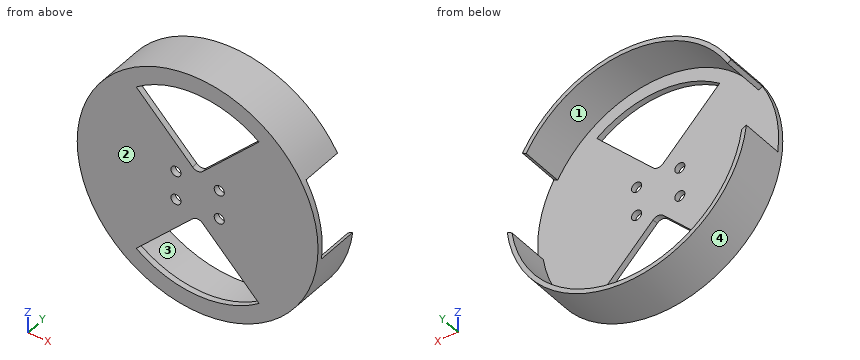
```python
from build123d import *

# Parameters (mm, degrees)
CROQUIS1_R              = 80.5
SALIENTE_EXTRUIR1_DEPTH = 4
CROQUIS2_R              = 83.5
CROQUIS2_R_2            = 80.5
EXTRUIR_L_MINA1_DEPTH   = 34
CORTAR_EXTRUIR1_START   = -30
CORTAR_EXTRUIR1_DEPTH   = 30
CORTAR_EXTRUIR3_DEPTH   = 4
CROQUIS6_R              = 3.5
CORTAR_EXTRUIR4_DEPTH   = 10


with BuildPart() as part:
    # Croquis1 → Saliente-Extruir1 (new body)
    with BuildSketch(Plane(origin=(0, 0, 0), x_dir=(1, 0, 0), z_dir=(0, 1, 0))):
        with Locations(Location((0, 0, 0), (0, 0, 270))):
            Circle(CROQUIS1_R)
    extrude(amount=SALIENTE_EXTRUIR1_DEPTH)

    # Croquis2 → Extruir-Lámina1 (add)
    with BuildSketch(Plane(origin=(0, 0, 0), x_dir=(1, 0, 0), z_dir=(0, 1, 0))):
        Circle(CROQUIS2_R)
        Circle(CROQUIS2_R_2, mode=Mode.SUBTRACT)
    extrude(amount=EXTRUIR_L_MINA1_DEPTH)

    # Croquis3 → Cortar-Extruir1 (cut)
    with BuildSketch(Plane(origin=(0, 34, 0), x_dir=(1, 0, 0), z_dir=(0, 1, 0)).offset(CORTAR_EXTRUIR1_START)):
        with BuildLine():
            Line((82.915347707, 9.8638286), (79.63686942, 11.756658922))
            ThreePointArc((79.63686942, 11.756658922), (80.283927371, 5.894150138), (80.5, 0))
            ThreePointArc((80.5, 0), (77.757029016, -20.834933131), (69.715045005, -40.25))
            Line((69.715045005, -40.25), (72.313121216, -41.75))
            ThreePointArc((72.313121216, -41.75), (80.654806495, -21.611390266), (83.5, 0))
            ThreePointArc((83.5, 0), (83.353708776, 4.940570133), (82.915347707, 9.8638286))
        make_face()
        with BuildLine():
            ThreePointArc((-69.715045005, -40.25), (-79.073837194, -15.085697577), (-79.63686942, 11.756658922))
            Line((-79.63686942, 11.756658922), (-82.915347707, 9.8638286))
            ThreePointArc((-82.915347707, 9.8638286), (-81.792213668, -16.801303023), (-72.313121216, -41.75))
            Line((-72.313121216, -41.75), (-69.715045005, -40.25))
        make_face()
    extrude(amount=CORTAR_EXTRUIR1_DEPTH, mode=Mode.SUBTRACT)

    # Croquis4 → Cortar-Extruir3 (cut)
    with BuildSketch(Plane.XZ):
        with BuildLine():
            Line((-42.603387144, 57.603387144), (-3.535533906, 18.535533906))
            ThreePointArc((-3.535533906, 18.535533906), (0, 17.071067812), (3.535533906, 18.535533906))
            Line((3.535533906, 18.535533906), (42.603387144, 57.603387144))
            ThreePointArc((42.603387144, 57.603387144), (0, 71.646345383), (-42.603387144, 57.603387144))
        make_face()
        with BuildLine():
            Line((-3.535533906, -18.535533906), (-42.603387144, -57.603387144))
            ThreePointArc((-42.603387144, -57.603387144), (0, -71.646345383), (42.603387144, -57.603387144))
            Line((42.603387144, -57.603387144), (3.535533906, -18.535533906))
            ThreePointArc((3.535533906, -18.535533906), (0, -17.071067812), (-3.535533906, -18.535533906))
        make_face()
    extrude(amount=-CORTAR_EXTRUIR3_DEPTH, mode=Mode.SUBTRACT)

    # Croquis6 → Cortar-Extruir4 (cut)
    with BuildSketch(Plane.XZ):
        with Locations(Location((-15, 10, 0), (0, 0, 270))):
            Circle(CROQUIS6_R)
        with Locations(Location((-15, -10, 0), (0, 0, 270))):
            Circle(CROQUIS6_R)
        with Locations(Location((15, 10, 0), (0, 0, 270))):
            Circle(CROQUIS6_R)
        with Locations(Location((15, -10, 0), (0, 0, 270))):
            Circle(CROQUIS6_R)
    extrude(amount=-CORTAR_EXTRUIR4_DEPTH, mode=Mode.SUBTRACT)


solid = part.part
```
CAD build for the part. Positions are in the model's coordinates, mm. Face numbers are marked on the shaded views. Give positions to 0.01 mm unless a question says otherwise; leave off trailing zeros. Loops run counter-clockwise (first coordinate to the right, second up) from the corner with the lowest first, then second, coordinate; pieces in that order, holes last. Notation, with made-up numbers: (-39.5, -20.5) -> (-6.5, -20.5) arc R13 ccw to (-6.5, -16.5) -> close; hole circle Ø11 at (3, -15). An arc over 180 degrees is marked (long way). Use a Markdown table: item, result.
1. Wall check: L1, parallel to X at y = 2.15, z = 10; L2, parallel to Y at x = -21.5, z = 33.5; L3, parallel to Z at x = -36, y = 16. Give the ranges that are in metal, low to high. Write a range as [from, to].
Check result:
| item | result |
|---|---|
| L1 | x = [-82.9, -18.5], [-11.5, 11.5], [18.5, 82.9] |
| L2 | y = [0, 4] |
| L3 | z = [-75.34, -72], [72, 75.34] |
2. Flat gauge pins, fed straight in: pin 1 (8 mm diameter, centred on y = 22, z = -58, fed in from +X); pin 2 (1 mm diameter, centred on x = -38.5, y = 6.5, fed in from +Z); pin 3 (5.5 mm diameter, centred on x = 15, z = -10, fed in from +Y); pin 4 (8 mm diameter, centred on x = -15, z = -10, fed in from +Y). Where does each tip first touch, or does it go through?
Check result:
| item | result |
|---|---|
| pin 1 | stops at x = 63.69 |
| pin 2 | stops at z = 74.35 |
| pin 3 | passes through |
| pin 4 | stops at y = 4 |
3. Slice it at B-B (x = 0). List the corners of the cut face in (y, z).
Check result:
| item | result |
|---|---|
| outline | (0, -83.5) -> (34, -83.5) -> (34, -80.5) -> (4, -80.5) -> (4, -71.65) -> (0, -71.65) -> close; (0, -17.07) -> (4, -17.07) -> (4, 17.07) -> (0, 17.07) -> close; (0, 71.65) -> (4, 71.65) -> (4, 80.5) -> (34, 80.5) -> (34, 83.5) -> (0, 83.5) -> close |
4. Slice it at C-C (z = -55). List the corners of the cut face in (x, y).
Check result:
| item | result |
|---|---|
| outline | (-62.83, 0) -> (-40, 0) -> (-40, 4) -> (-58.78, 4) -> (-58.78, 34) -> (-62.83, 34) -> close; (40, 0) -> (62.83, 0) -> (62.83, 34) -> (58.78, 34) -> (58.78, 4) -> (40, 4) -> close |
5. Slice it at A-A (y = 19). List the corners of the cut face in (x, z), plus the area to 3 significant figures.
Check result:
| item | result |
|---|---|
| outline | (-82.92, -9.86) arc R83.5 ccw to (82.92, -9.86) -> (79.64, -11.76) arc R80.5 cw to (-79.64, -11.76) -> close; (-72.31, 41.75) -> (-69.72, 40.25) arc R80.5 cw to (69.72, 40.25) -> (72.31, 41.75) arc R83.5 ccw to start |
| area | 1,220 mm^2 |
6. Mould opens along Z. For the marked faces 1, 2, 3 and 4 say: pulls with the +Z half, pulls with the -Z half, needs draft (parallel to the pull), parting line crosses it, or undercut.
Check result:
| item | result |
|---|---|
| face 1 | undercut |
| face 2 | needs draft |
| face 3 | undercut |
| face 4 | parting line crosses it |
7. Slice it at D-D (z = 10). List the corners of the cut face in (x, y).
Check result:
| item | result |
|---|---|
| outline | (-82.9, 0) -> (-18.5, 0) -> (-18.5, 4) -> (-82.9, 4) -> close; (-11.5, 0) -> (11.5, 0) -> (11.5, 4) -> (-11.5, 4) -> close; (18.5, 0) -> (82.9, 0) -> (82.9, 4) -> (18.5, 4) -> close |
